Geometry: final body of the model. Coordinates: model frame, mm. A direction names the side the tool comes from. Give positions to 0.01 mm unless a question says otherwise; leave off trailing zeros. Write each loop counter-clockwise with the first axis right and the second up, starting at its lowest first coordinate (ties: lowest second). Pieces come first, ordered by that corner, then holes. Notation, with made-up numbers: (-4, -18.5) - (6, -18.5) arc R12 ccw to (6, -13.5) - close; hole circle Ø6 at (36, 78). An arc over 180 degrees is marked (long way). Return JSON: item names as keys, results as strings.
Autodesk Inventor part; units mm, degrees
ref_plane "YZ Plane" through (0, 0, 0) normal (1, 0, 0) x (0, 1, 0)
ref_plane "XZ Plane" through (0, 0, 0) normal (0, 1, 0) x (-1, 0, 0)
ref_plane "XY Plane" through (0, 0, 0) normal (0, 0, 1) x (1, 0, 0)
sketch "Boceto1" plane through (0, 0, 0) normal (0, 1, 0) x (-1, 0, 0)
  circle A0 centre (0, 0) radius 9.325
  dimension "d0" = 18.65
extrude "Extrusión1" add sketch "Boceto1" along normal blind 20
sketch "Boceto2" plane through (0, 20, 0) normal (0, 1, 0) x (1, 0, 0)
  circle A0 centre (0, 0) radius 4.625
  dimension "d3" = 9.25
extrude "Extrusión2" add sketch "Boceto2" along normal blind 9
sketch "Boceto3" plane through (0, 29, 0) normal (0, 1, 0) x (1, 0, 0)
  circle A0 centre (0, 0) radius 4.625
hole "Agujero1" at (0, 29, 0) direction (0, -1, 0) diameter 6.5 end through all
chamfer "Chaflán1" distance 2 angle 45 1 edges at (9.325, 0, 0)
chamfer "Chaflán2" distance 1 angle 45 1 edges at (-4.625, 29, 0)
fillet "Empalme1" radius 1 1 edges at (-4.625, 20, 0)
equation "\"d30\" = 0.125 * Sketch4_Pitch"
equation "\"Sketch4_Pitch\" = 1.5"
equation "\"d32\" = 60deg"
properties part number "OutputFile"
Q1. Section query D-D, the plane y = 22. Return the cut outline in (x, z) (3 decimals).
Answer key:
{"outline": "circle Ø9.25 at (0, 0); hole circle Ø6.5 at (0, 0)"}
Q2. Section query C-C, the plane y = 9.75. Return the cut outline in (x, z) (3 decimals), plus the area to 3 significant figures.
Answer key:
{"outline": "circle Ø18.65 at (0, 0); hole circle Ø6.5 at (0, 0)", "area": "240 mm^2"}
Q3. Pin query (flat end, axial travel): P1, Ø3, axis at x = -7, y = 10, coming from the +Z side; P2, Ø8, axis at y = 4, z = -1, coming from the -X side (3 decimals); P3, Ø1.5, axis at x = 2, z = 7, coming from the +Y side; P4, Ø1, axis at x = -3.5, y = 14, coming from the +Z side. Return the tip coordinate at first contact, or that it passes through.
Answer key:
{"P1": "stops at z = 7.53", "P2": "stops at x = -9.325", "P3": "stops at y = 20", "P4": "stops at z = 8.83"}
Q4. Section query A-A, the plane x = 0. Return the cut outline in (y, z) (3 decimals).
Answer key:
{"outline": "(0, -7.325) - (2, -9.325) - (20, -9.325) - (20, -5.625) arc R1 cw to (21, -4.625) - (28, -4.625) - (29, -3.625) - (29, -3.25) - (0, -3.25) - close; (0, 3.25) - (29, 3.25) - (29, 3.625) - (28, 4.625) - (21, 4.625) arc R1 cw to (20, 5.625) - (20, 9.325) - (2, 9.325) - (0, 7.325) - close"}
Q5. Material intervals for probe 1 along Z at (x, y) = (0, 12.25) (3 decimals); probe 2 along Z at (x, y) = (0, 22.5) (3 decimals); probe 3 along Y at (x, z) = (5.75, 2.5), sorted ascending. Write a range as [from, to].
Answer key:
{"probe 1": "z = [-9.325, -3.25], [3.25, 9.325]", "probe 2": "z = [-4.625, -3.25], [3.25, 4.625]", "probe 3": "y = [0, 20]"}
Q6. Section query B-B, the plane z = 0. Return the cut outline in (x, y) (3 decimals).
Answer key:
{"outline": "(-9.325, 2) - (-7.325, 0) - (-3.25, 0) - (-3.25, 29) - (-3.625, 29) - (-4.625, 28) - (-4.625, 21) arc R1 cw to (-5.625, 20) - (-9.325, 20) - close; (3.25, 0) - (7.325, 0) - (9.325, 2) - (9.325, 20) - (5.625, 20) arc R1 cw to (4.625, 21) - (4.625, 28) - (3.625, 29) - (3.25, 29) - close"}
Q7. Mould query, pull axis Z, two halves, no side actions, for faces 3 (the flat face through (-3, 0, -2)), 4 (the cylindrical face through (1.978, 14.297, -2.579)), 5 (the cylindrical face through (7.4, 10.874, 5.674)). Classes: pulls with the +Z half, pulls with the -Z half, needs draft (parallel to the pull), parting line crosses it, or undercut.
Answer key:
{"face 3": "needs draft", "face 4": "undercut", "face 5": "parting line crosses it"}
Q8. Set-up query: faces 1 (the conical face through (7.443, 0.125, 0.328)), 2 (the cylindrical face through (-1.003, 24.451, -4.515)). Return all of +Z, -Z, +X, -X, +Y, -Y with unobstructed straight access to the full face (end or side cutting, diameter ignored); none if empty.
Answer key:
{"face 1": "-Y", "face 2": "+Y"}
